Could you check a few things on this model? Use its own coordinates, in mm. A direction names the side the tool comes from. Give positions to 0.01 mm unless a question says otherwise; leave off trailing zeros. Loops run counter-clockwise (first coordinate to the right, second up) from the corner with the lowest first, then second, coordinate; pieces in that order, holes last. Notation, with made-up numbers: (33, -3) - (43, -3) arc R14 ccw to (43, 24) - close; hole circle Ø2 at (39, 87.25). An arc over 180 degrees is marked (long way). Write each question's results on one line, items separated by ' | '. Start each with the question number.
1) If we mould it in two halves opening along X, with no side actions, what happens to faces 1 (the face through (-30, 39.4, 0.4)), 2 (the face through (-63, 37, -34)), 3 (the face through (-5, 32, 0))? For each: +X half, -X half, draft (parallel to the pull), parting line (faces both ways), or undercut.
2) If I drill on probe 1 along X at (y, z) = (40.5, -33); probe 2 along Z at (x, y) = (34.5, 59); probe 3 along X at (y, z) = (48, -43), over which ranges is the centre line in solid material (lowest first)? Write a range as [from, to].
3) I want a section at B-B, the plane z = -29. Write out the boundary of the cut face in (x, y).
4) I want a section at C-C, the plane x = -27. Write out the boundary of the cut face in (y, z), and give its area (3 significant figures).
5) I'm going to push flat-ended pins straight in: pin 1 (16.5 mm diameter, centred on x = -1, y = 39.5, fed in from -Z); pin 2 (0.6 mm diameter, centred on x = -26.5, z = -14, fed in from +Y); pin 3 (8 mm diameter, centred on y = 38, z = -10.5, fed in from -X); pin 4 (0.8 mm diameter, centred on y = 70.5, z = -16.5, fed in from +X). Where does each tip first touch, or does it pass through?
6) I want a section at D-D, the plane z = -44.5. Write out the boundary of the cut face in (x, y).
7) On a 3-axis mill with a long thin cutter (end or side, diameter ignored), from which of +Z, -Z, +X, -X, +Y, -Y can I reach the whole of each face in a straight line? I mean faces 4 (the face through (-5, 2, -14)), 5 (the face through (-25.18, 66.4, -7.34)), 6 (the face through (-43, 37, -19)). Say none if no direction works.
8) I want a section at A-A, the plane y = 38. Count the separate pieces of the cut face and the enclosed holes in it, and give its area (3 significant figures).
from build123d import *

# Parameters (mm, degrees)
BOSS_EXTRUDE1_DEPTH      = 30
FILLET1_R                = 5
SKETCH2_W                = 11
SKETCH2_H                = 68.4
CUT_EXTRUDE1_DEPTH       = 17
BOSS_EXTRUDE3_DEPTH      = 2
BOSS_EXTRUDE4_DEPTH      = 32
SKETCH4_W                = 2
SKETCH4_H                = 70
BOSS_EXTRUDE5_DEPTH      = 18.2
BOSS_EXTRUDE6_DEPTH      = 10
BOSS_EXTRUDE6_DEPTH_BACK = 10
BOSS_EXTRUDE7_START      = 20
BOSS_EXTRUDE7_DEPTH      = 10
BOSS_EXTRUDE8_START      = -30
BOSS_EXTRUDE8_DEPTH      = 10
CHAMFER1_SIZE            = 2
CUT_EXTRUDE2_REACH       = 134.608
SKETCH6_R                = 6


with BuildPart() as part:
    # Sketch1 → Boss-Extrude1 (new body)
    with BuildSketch(Plane(origin=(0, 0, 0), x_dir=(0, 0, -1), z_dir=(1, 0, 0))):
        with BuildLine():
            ThreePointArc((-2, 58.9), (7.5, 68.4), (17, 58.9))
            Line((17, 58.9), (17, 0))
            Line((17, 0), (15, 0))
            Line((15, 0), (15, 58.9))
            ThreePointArc((15, 58.9), (7.5, 66.4), (0, 58.9))
            Line((0, 58.9), (0, 0))
            Line((0, 0), (-2, 0))
            Line((-2, 0), (-2, 58.9))
        make_face()
        with BuildLine():
            Line((-2, 0), (0, 0))
            Line((0, 0), (0, 4))
            Line((0, 4), (0, 58.9))
            ThreePointArc((0, 58.9), (2.196699141, 64.203300859), (7.5, 66.4))
            Line((7.5, 66.4), (7.5, 68.4))
            ThreePointArc((7.5, 68.4), (0.782485579, 65.617514421), (-2, 58.9))
            Line((-2, 58.9), (-2, 0))
        make_face()
        Polygon((0, 4), (0, 0), (2, 4), align=None)
        Polygon((15, 0), (15, 4), (13, 4), align=None)
        with BuildLine():
            Line((17, 68.4), (7.5, 68.4))
            ThreePointArc((7.5, 68.4), (14.217514421, 65.617514421), (17, 58.9))
            Line((17, 58.9), (17, 68.4))
        make_face()
        with BuildLine():
            Line((-2, 68.4), (-2, 58.9))
            ThreePointArc((-2, 58.9), (0.782485579, 65.617514421), (7.5, 68.4))
            Line((7.5, 68.4), (-2, 68.4))
        make_face()
    extrude(amount=-BOSS_EXTRUDE1_DEPTH)

    # Fillet1
    fillet1_edges = [part.edges().sort_by_distance(p)[0] for p in [
        (-15, 68.4, 2),
    ]]
    fillet(fillet1_edges, radius=FILLET1_R)

    # Sketch2 → Cut-Extrude1 (cut)
    with BuildSketch(Plane.XY.offset(2)):
        with Locations((-15, 34.2)):
            Rectangle(SKETCH2_W, SKETCH2_H)
    extrude(amount=-CUT_EXTRUDE1_DEPTH, mode=Mode.SUBTRACT)

    # Sketch3 → Boss-Extrude3 (add)
    with BuildSketch(Plane(origin=(0, 0, -17), x_dir=(-1, 0, 0), z_dir=(0, 0, -1))):
        Polygon((-33, 2), (0, 2), (0, 0), (65, 0), (65, 72), (-33, 72), align=None)
    extrude(amount=BOSS_EXTRUDE3_DEPTH)

    # Sketch3<3> → Boss-Extrude4 (add)
    with BuildSketch(Plane(origin=(0, 0, -17), x_dir=(-1, 0, 0), z_dir=(0, 0, -1))):
        Polygon((65, 72), (63, 72), (63, 2), (-33, 2), (-33, 72), (-35, 72), (-35, 0), (65, 0), align=None)
    extrude(amount=BOSS_EXTRUDE4_DEPTH)

    # Sketch4 → Boss-Extrude5 (add)
    with BuildSketch(Plane(origin=(0, 0, -19), x_dir=(-1, 0, 0), z_dir=(0, 0, -1))):
        with Locations((23, 37)):
            Rectangle(SKETCH4_W, SKETCH4_H)
    extrude(amount=BOSS_EXTRUDE5_DEPTH)

    # Sketch5 → Boss-Extrude6 (add, two sides: drawn at the far end of the back side and taken through both)
    with BuildSketch(Plane.ZY.offset(15).offset(-BOSS_EXTRUDE6_DEPTH_BACK)):
        with BuildLine():
            Line((-48.8, 0), (-46.8, 0))
            ThreePointArc((-46.8, 0), (-47.8, -1), (-48.8, 0))
        make_face()
    extrude(amount=BOSS_EXTRUDE6_DEPTH + BOSS_EXTRUDE6_DEPTH_BACK)

    # Sketch5<3> → Boss-Extrude7 (add)
    with BuildSketch(Plane.ZY.offset(15).offset(BOSS_EXTRUDE7_START)):
        with BuildLine():
            ThreePointArc((-17, 72), (-16, 71), (-17, 70))
            Line((-17, 70), (-17, 72))
        make_face()
    extrude(amount=BOSS_EXTRUDE7_DEPTH)

    # Sketch5<4> → Boss-Extrude8 (add)
    with BuildSketch(Plane.ZY.offset(15).offset(BOSS_EXTRUDE8_START)):
        with BuildLine():
            ThreePointArc((-17, 72), (-16, 71), (-17, 70))
            Line((-17, 70), (-17, 72))
        make_face()
    extrude(amount=BOSS_EXTRUDE8_DEPTH)

    # Chamfer1
    chamfer1_edges = [part.edges().sort_by_distance(p)[0] for p in [
        (-30, 34.2, -17),
        (0, 34.2, -17),
    ]]
    chamfer(chamfer1_edges, length=CHAMFER1_SIZE - 0.0001)  # a hair under: the kernel refuses the full size

    # Sketch6 → Cut-Extrude2 (cut, up to next)
    with BuildSketch(Plane(origin=(35, 0, 0), x_dir=(0, 0, -1), z_dir=(1, 0, 0)), mode=Mode.PRIVATE) as cut_extrude2_sk1:
        with Locations(Location((29, 59, 0), (0, 0, 90))):
            Circle(SKETCH6_R)
    cut_extrude2_tool1 = extrude(cut_extrude2_sk1.sketch, amount=-CUT_EXTRUDE2_REACH, mode=Mode.PRIVATE) & part.part
    add(cut_extrude2_tool1.solids().sort_by_distance((35, 59, -29))[0], mode=Mode.SUBTRACT)


solid = part.part
Answers:
1) face 1: -X half | face 2: undercut | face 3: draft
2) probe 1: x = [-65, -63], [-24, -22], [33, 35] | probe 2: z = [-49, -35], [-23, -17] | probe 3: x = [-65, -63], [33, 35]
3) outline: (-65, 0) - (35, 0) - (35, 53) - (33, 53) - (33, 2) - (-22, 2) - (-22, 72) - (-24, 72) - (-24, 2) - (-63, 2) - (-63, 72) - (-65, 72) - close; (33, 65) - (35, 65) - (35, 72) - (33, 72) - close
4) outline: (0, -49) - (2, -49) - (2, -19) - (72, -19) - (72, -17) - (68.4, -17) - (68.4, -3) arc R5 ccw to (63.4, 2) - (0, 2) - (0, 0) - (4, -2) - (4, 0) - (58.9, 0) arc R7.5 cw to (58.9, -15) - (4, -15) - (4, -13) - (0, -15) - close | area: 534 mm2
5) pin 1: stops at z = -19 | pin 2: stops at y = 68.4 | pin 3: passes through | pin 4: stops at x = 15
6) outline: (-65, 0) - (35, 0) - (35, 72) - (33, 72) - (33, 2) - (-63, 2) - (-63, 72) - (-65, 72) - close
7) face 4: +X, -X, -Y | face 5: +X, -X | face 6: -Z, +Y
8) separate pieces: 3 | enclosed holes: 0 | area: 458 mm2
